Can you work these out from the drawing? Everything is in mm from the part's minimum corner. A direction names the side the tool comes from. Give positions to 0.01 mm unless a question says otherwise; leave off trailing zeros. Order: outer loops, then holes, each group sorted by start corner. A loop starts at its lowest first (then second) coordinate and runs counter-clockwise, first axis right, second up. Notation, with made-up numbers: (85, 76) - (135, 76) arc R14 cw to (135, 86) - close; hole circle Ø11 at (-3.75, 74). An arc over 180 degrees is marked (long way). Answer as a JSON object with one key per item and string values.
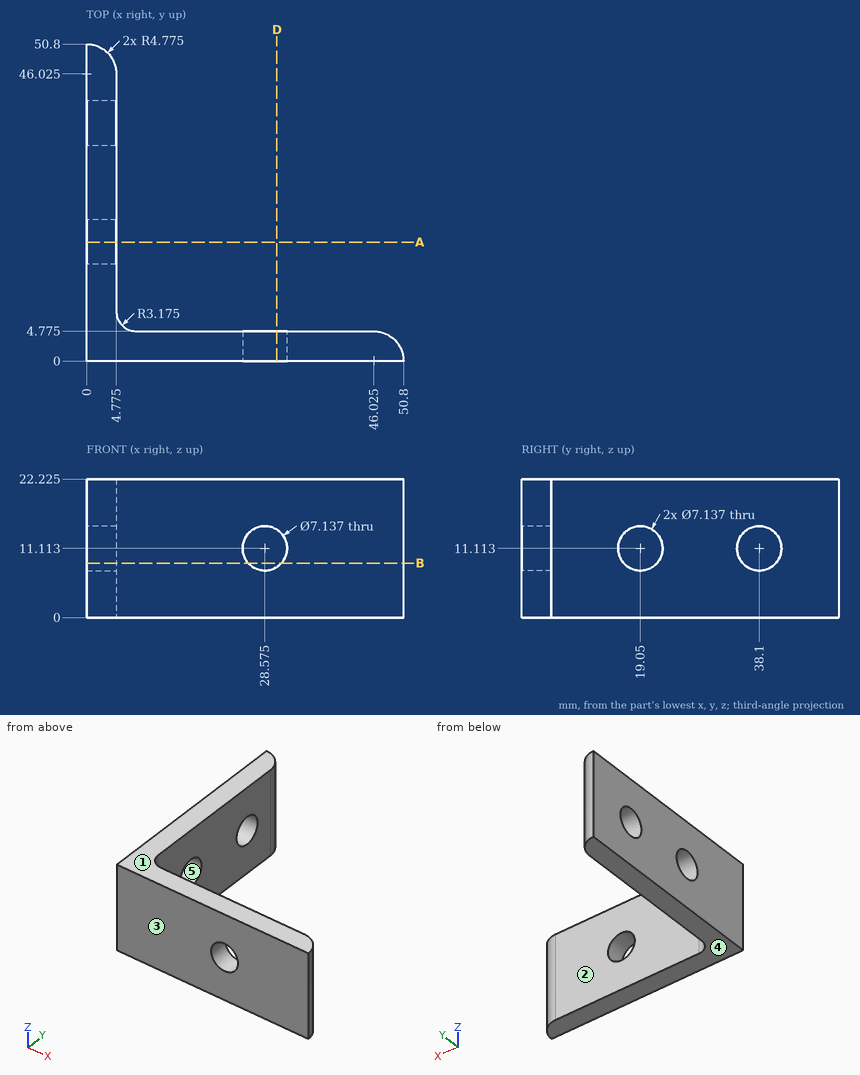
Q1. I'm going to push flat-ended pins straight in: pin 1 Ø11 at (x, z) = (24, 11.5) entering from +Y (1 decimal); pin 2 Ø6.5 at (y, z) = (38.1, 11.11) entering from +X; pin 3 Ø5 at (y, z) = (33, 15) entering from +X (1 decimal). Where does each tip first touch, or does it pass through?
Recorded:
{"pin 1": "stops at y = 4.8", "pin 2": "passes through", "pin 3": "stops at x = 4.8"}
Q2. We'd pull the mould along Y, two halves only. Please class the marked faces 3, 4 and 5: released by +Y, released by -Y, zero draft, split by the parting line, or undercut.
Recorded:
{"face 3": "released by -Y", "face 4": "zero draft", "face 5": "undercut"}
Q3. If we section it at D-D, the plane x = 30.5: Please give me the cut outline in (y, z) (1 decimal).
Recorded:
{"outline": "(0, 0) - (4.8, 0) - (4.8, 8.1) - (0, 8.1) - close; (0, 14.1) - (4.8, 14.1) - (4.8, 22.2) - (0, 22.2) - close"}
Q4. I need wall thicknesses on L1, parallel to Z at x = 1.75, y = 38.1 (1 decimal); L2, parallel to Y at x = 46, z = 7.5 (1 decimal). Which ranges of each line are inside material? Lowest first, please.
Recorded:
{"L1": "z = 0 to 7.5, 14.7 to 22.2", "L2": "y = 0 to 4.8"}
Q5. Which directions (+Z, -Z, +X, -X, +Y, -Y) give clear straight access to the entire face, cutting with the end or side of a thin tool? Please do the marked faces 1 and 2.
Recorded:
{"face 1": "+Z, +X, -X, +Y, -Y", "face 2": "+Z, -Z, +X, +Y"}
Q6. If we section it at A-A, the plane y = 19.05: Please give me the cut outline in (x, z) (1 decimal).
Recorded:
{"outline": "(0, 0) - (4.8, 0) - (4.8, 7.5) - (0, 7.5) - close; (0, 14.7) - (4.8, 14.7) - (4.8, 22.2) - (0, 22.2) - close"}
Q7. If we section it at B-B, the plane z = 8.75: Count the separate pieces of the cut face and the enclosed holes in it, then the cut area to 3 significant figures.
Recorded:
{"separate pieces": "4", "enclosed holes": "0", "area": "378 mm^2"}
